CAD build for the part. Positions are in the model's coordinates, mm. Face numbers are marked on the shaded views. A direction names the side the tool comes from. Round coordinates to 2 decimals unless told otherwise and drop trailing zeros. Order: outer loops, then holes, each group sorted by start corner. A loop starts at its lowest first (then second) coordinate and runs counter-clockwise, first axis right, second up. Notation, with made-up numbers: M -28.75,84.5 L 6.25,84.5 A12 cw 6.25,98.5 Z; hole C -33.75,4.5 d11. An arc over 180 degrees is marked long. Put each result on its own line as item: value.
```python
from build123d import *

# Parameters (mm, degrees)
SKETCH2_W           = 240
SKETCH2_H           = 140
BOSS_EXTRUDE1_DEPTH = 1
SKETCH3_W           = 240
SKETCH3_H           = 140
SKETCH3_W_2         = 236
SKETCH3_H_2         = 136
BOSS_EXTRUDE2_DEPTH = 20
SKETCH4_W           = 236
SKETCH4_H           = 136
BOSS_EXTRUDE3_DEPTH = 4
SKETCH6_W           = 11
SKETCH6_H           = 56
CUT_EXTRUDE2_DEPTH  = 3
FILLET1_R           = 5
FILLET2_R           = 5
FILLET3_R           = 0.5
FILLET4_R           = 1


with BuildPart() as part:
    # Sketch2 → Boss-Extrude1 (new body)
    with BuildSketch(Plane(origin=(0, 0, 0), x_dir=(1, 0, 0), z_dir=(0, 1, 0))):
        Rectangle(SKETCH2_W, SKETCH2_H)
    extrude(amount=BOSS_EXTRUDE1_DEPTH)

    # Sketch3 → Boss-Extrude2 (add)
    with BuildSketch(Plane(origin=(0, 1, 0), x_dir=(1, 0, 0), z_dir=(0, 1, 0))):
        Rectangle(SKETCH3_W, SKETCH3_H)
        Rectangle(SKETCH3_W_2, SKETCH3_H_2, mode=Mode.SUBTRACT)
    extrude(amount=BOSS_EXTRUDE2_DEPTH)

    # Sketch4 → Boss-Extrude3 (add)
    with BuildSketch(Plane(origin=(0, 21, 0), x_dir=(1, 0, 0), z_dir=(0, 1, 0))):
        Polygon((-125, 80), (-120, 80), (-120, 75), (120, 75), (120, -75), (-120, -75), (-120, -80), (-125, -80), (-125, -30), (-135, -30), (-135, 30), (-125, 30), align=None)
        Rectangle(SKETCH4_W, SKETCH4_H, mode=Mode.SUBTRACT)
    extrude(amount=BOSS_EXTRUDE3_DEPTH)

    # Sketch6 → Cut-Extrude2 (cut)
    with BuildSketch(Plane.XZ.offset(-21)):
        with Locations((-127.5, 0)):
            Rectangle(SKETCH6_W, SKETCH6_H)
    extrude(amount=-CUT_EXTRUDE2_DEPTH, mode=Mode.SUBTRACT)

    # Fillet1
    fillet1_edges = [part.edges().sort_by_distance(p)[0] for p in [
        (0, 1, 68),
        (118, 1, 0),
        (0, 1, -68),
        (-118, 13, 68),
        (118, 13, 68),
        (118, 13, -68),
        (-118, 13, -68),
        (-120, 0, 0),
    ]]
    fillet(fillet1_edges, radius=FILLET1_R)

    # Fillet2
    fillet2_edges = [part.edges().sort_by_distance(p)[0] for p in [
        (2.5, 0, 70),
        (-118.535533906, 1.464466094, 70),
        (-118.535533906, 1.464466094, -70),
        (2.5, 0, -70),
        (120, 0, 0),
        (120, 10.5, 70),
        (-120, 13, 70),
        (-120, 13, -70),
        (120, 10.5, -70),
    ]]
    fillet(fillet2_edges, radius=FILLET2_R)

    # Fillet3
    fillet3_edges = [part.edges().sort_by_distance(p)[0] for p in [
        (-125, 21, 55),
        (-122.5, 21, 80),
        (-125, 23, 80),
        (-120, 21, 77.5),
        (-120, 23, 80),
        (0, 21, 75),
        (-120, 23, 75),
        (120, 21, 67.5),
        (120, 21, -67.5),
        (120, 23, 75),
        (0, 21, -75),
        (120, 23, -75),
        (-120, 21, -77.5),
        (-120, 23, -75),
        (-122.5, 21, -80),
        (-120, 23, -80),
        (-125, 21, -55),
        (-125, 23, -80),
    ]]
    fillet(fillet3_edges, radius=FILLET3_R)

    # Fillet4
    fillet4_edges = [part.edges().sort_by_distance(p)[0] for p in [
        (-135, 23, -30),
        (-135, 23, 30),
        (-122, 24, 0),
        (-122, 22.5, 28),
        (-127.5, 24, -28),
        (-122, 22.5, -28),
        (-133, 24, 0),
        (-133, 22.5, -28),
        (-127.5, 24, 28),
        (-133, 22.5, 28),
    ]]
    fillet(fillet4_edges, radius=FILLET4_R)


solid = part.part
```
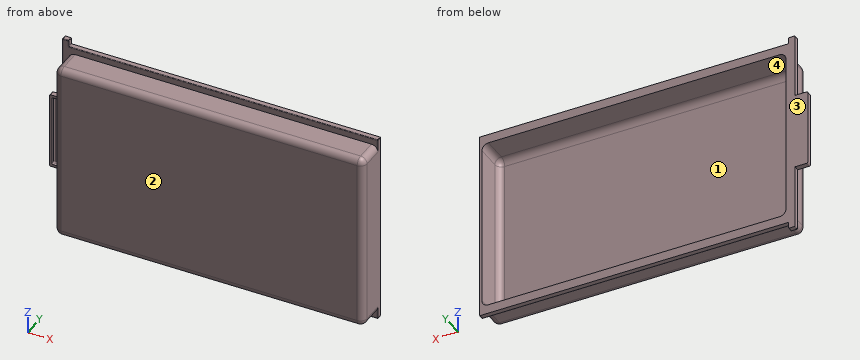
Item 1: Band-saw the part on C-C on x = -1.5. Give the cut face in (y, z).
Answers below:
outline: M 0,-65 A5 ccw 5,-70 L 21,-70 L 21,-74.5 A0.5 ccw 21.5,-75 L 25,-75 L 25,-68 L 6,-68 A5 cw 1,-63 L 1,63 A5 cw 6,68 L 25,68 L 25,75 L 21.5,75 A0.5 ccw 21,74.5 L 21,70 L 5,70 A5 ccw 0,65 Z
Item 2: Mould opens along Z. For the marked faces 3 and 4 say: pulls with the +Z half, pulls with the -Z half, needs draft (parallel to the pull), parting line crosses it, or undercut.
Answers below:
face 3: needs draft
face 4: undercut
Item 3: Band-saw the part on B-B on y = 13.75. Give the cut face in (x, z).
Answers below:
outline: M -120,-65 A5 ccw -115,-70 L 115,-70 A5 ccw 120,-65 L 120,65 A5 ccw 115,70 L -115,70 A5 ccw -120,65 Z; hole M -118,-63 A5 ccw -113,-68 L 113,-68 A5 ccw 118,-63 L 118,63 A5 ccw 113,68 L -113,68 A5 ccw -118,63 Z
Item 4: Tool access for the marked faces 1 and 2: list every direction of +Z, -Z, +X, -X, +Y, -Y with a clear straight run to the whole face (end or side of a thin tool).
Answers below:
face 1: +Y
face 2: +Z, -Z, +X, -X, -Y
Item 5: Pin check, flat tips, straight feed: P1, Ø10, axis at x = 27.5, z = -32.5, coming from the +Y side; P2, Ø3, axis at x = -131.5, y = 23.5, coming from the +Z side; P3, Ø3, axis at x = 6.5, y = 23, coming from the +Z side. Stop position of each tip, or through.
Answers below:
P1: y = 1
P2: z = 30
P3: z = 75
Item 6: Probe line 1 along X through (y, z) = (17, 39); line 2 along Z through (x, y) = (-99.5, 22.5); line 3 along X through (y, z) = (22.75, -46). List the from-to ranges inside material, lowest first. Write a range as [from, to].
Answers below:
line 1: [-120, -118], [118, 120]
line 2: [-75, -68], [68, 75]
line 3: [-125, -118], [118, 120]
